Here's how the part is built. I have some questions about the finished solid (model axes, mm). A direction names the side the tool comes from. Coordinates: 2 decimals unless noted, no trailing zeros. Loops run counter-clockwise (first coordinate to the right, second up) from the corner with the lowest first, then second, coordinate; pieces in that order, holes last.
Autodesk Inventor part; units mm, degrees
ref_plane "YZ Plane" through (0, 0, 0) normal (1, 0, 0) x (0, 1, 0)
ref_plane "XZ Plane" through (0, 0, 0) normal (0, 1, 0) x (-1, 0, 0)
ref_plane "XY Plane" through (0, 0, 0) normal (0, 0, 1) x (1, 0, 0)
sketch "Sketch1" plane through (0, 0, 0) normal (0, 0, 1) x (1, 0, 0)
  line L0 (0, 1.5) -> (3.75, 1.5)
  line L1 (3.75, 1.5) -> (3.75, -1)
  line L2 (3.75, -1) -> (2.25, -1)
  line L3 (2.25, -1) -> (2.25, -1.5)
  line L4 (2.25, -1.5) -> (0, -1.5)
  line L5 (0, 1.5) -> (0, -1.5)
  point P0 (0, 0)
  point P1 (0, 0)
  dimension "d0" = 2.5
  dimension "d1" = 0.5
  dimension "d2" = 3.75
  dimension "d3" = 2.25
revolve "Revolution1" add sketch "Sketch1" angle 360 about axis through (0, 1.5, 0) along (0, -1, 0)
sketch "Sketch2" plane through (0, -1.5, 0) normal (0, -1, 0) x (1, 0, 0)
  point P0 (0, 0)
  point P1 (0, 0)
hole "Hole1" at (0, -1.5, 0) direction (0, 1, 0) diameter 2.459 end through all
chamfer "Chamfer1" distance 0.4 angle 45 2 edges at (0, 1.5, 1.2295) (-3.75, 1.5, 0)
properties part number "RPS Basic M3 Weld Nut" material "Stainless Steel"
Q1. Suppose I cut it at C-C on y = -1.25. Write out the boundary of the cut face in (x, z), and give its area (3 significant figures).
Q2. Please list where these lines run through material, in increasing order: probe 1 along Z at (x, y) = (0, 0.45); probe 2 along Y at (x, z) = (-1.75, 2); probe 3 along Z at (x, y) = (0.5, 0.8).
Q3. We'd pull the mould along X, two halves only. Please class faces 1 (the cylindrical face through (-0.29, -1.25, 2.23)), 2 (the flat face through (-2, 1.5, -1)), 3 (the cylindrical face through (0.748, -0.182, 0.976)): pulls with the +X half, pulls with the -X half, needs draft (parallel to the pull), parting line crosses it, or undercut.
Q4. Will this pin go through, and if not, where does the flat tip stop? P1, Ø1.5, axis at x = -2, y = 0, coming from the +Z side.
Q5. Suppose I cut it at B-B on x = 0. Write out the boundary of the cut face in (y, z), and give its area (3 significant figures).
Q6. Suppose I cut it at A-A on z = 0. Write out the boundary of the cut face in (x, y).
Q7. For faces 4 (the flat face through (1, -1.5, -1)), 5 (the flat face through (2, -1, -2)), which set-ups out of +Z, -Z, +X, -X, +Y, -Y let a thin tool reach every point of the face, with its end or its side?
Q8. Suppose I cut it at D-D on y = 0.85. Write out the boundary of the cut face in (x, z), and give its area (3 significant figures).
Check values:
1. outline: circle Ø4.5 at (0, 0); hole circle Ø2.46 at (0, 0)
1. area: 11.2 mm2
2. probe 1: z = -3.75 to -1.23, 1.23 to 3.75
2. probe 2: y = -1 to 1.5
2. probe 3: z = -3.72 to -1.12, 1.12 to 3.72
3. face 1: parting line crosses it
3. face 2: needs draft
3. face 3: undercut
4. P1: stops at z = 3.54
5. outline: (-1.5, -2.25) - (-1, -2.25) - (-1, -3.75) - (1.1, -3.75) - (1.5, -3.35) - (1.5, -1.63) - (1.1, -1.23) - (-1.5, -1.23) - close; (-1.5, 1.23) - (1.1, 1.23) - (1.5, 1.63) - (1.5, 3.35) - (1.1, 3.75) - (-1, 3.75) - (-1, 2.25) - (-1.5, 2.25) - close
5. area: 13.3 mm2
6. outline: (-3.75, -1) - (-2.25, -1) - (-2.25, -1.5) - (-1.23, -1.5) - (-1.23, 1.1) - (-1.63, 1.5) - (-3.35, 1.5) - (-3.75, 1.1) - close; (1.23, -1.5) - (2.25, -1.5) - (2.25, -1) - (3.75, -1) - (3.75, 1.1) - (3.35, 1.5) - (1.63, 1.5) - (1.23, 1.1) - close
7. face 4: +Z, -Z, +X, -X, -Y
7. face 5: -Y
8. outline: circle Ø7.5 at (0, 0); hole circle Ø2.46 at (0, 0)
8. area: 39.4 mm2
